For this review, take the finished solid that the model builds, in its own axes (mm). A direction names the side the tool comes from. Give positions to 0.01 mm unless a question says otherwise; leave off trailing zeros. Order: outer loops, then holes, each group sorted by start corner. A loop starts at its lowest first (then second) coordinate and runs counter-clockwise, first axis right, second up. Notation, with made-up numbers: (88, 75.25) -> (122, 75.25) arc R27 cw to (122, 92.25) -> close; hole circle Ø11 at (24.5, 31.25). An arc over 180 degrees is marked (long way). One line per item, written item: value. Start each with the question number.
from build123d import *

# Parameters (mm, degrees)
SKETCH2_R           = 4.2
BOSS_EXTRUDE1_DEPTH = 100
FILLET1_R           = 5


with BuildPart() as part:
    # Sketch2 → Boss-Extrude1 (new body)
    with BuildSketch(Plane.XY):
        with BuildLine():
            Line((15.440624277, -4.881535018), (15.440624277, -0.681535018))
            ThreePointArc((15.440624277, -0.681535018), (3.240624277, 11.518464982), (-8.959375723, -0.681535018))
            Line((-8.959375723, -0.681535018), (-8.959375723, -4.881535018))
            Line((-8.959375723, -4.881535018), (-43.959375723, -4.881535018))
            Line((-43.959375723, -4.881535018), (-43.959375723, -10.881535018))
            Line((-43.959375723, -10.881535018), (50.440624277, -10.881535018))
            Line((50.440624277, -10.881535018), (50.440624277, -4.881535018))
            Line((50.440624277, -4.881535018), (15.440624277, -4.881535018))
        make_face()
        with Locations((3.240624277, -0.681535018)):
            Circle(SKETCH2_R, mode=Mode.SUBTRACT)
    extrude(amount=BOSS_EXTRUDE1_DEPTH)

    # Fillet1
    fillet1_edges = [part.edges().sort_by_distance(p)[0] for p in [
        (-8.959375723, -4.881535018, 50),
        (15.440624277, -4.881535018, 50),
    ]]
    fillet(fillet1_edges, radius=FILLET1_R)


solid = part.part
Q1. Take a section at A-A (x = 0.5). State the section outline as (y, z) points.
Q2. Take a section at B-B (y = 1.75). State the section outline as (x, z) points.
Q3. Mouldability with a two-part tool opening along Y and no side actions: class faces 1 (the cylindrical face through (-0.09, -3.24, 49.3)), 2 (the flat face through (36, -4.882, 49)), 3 (the flat face through (3, -10.882, 49)) as pulls with the +Y half, pulls with the -Y half, needs draft (parallel to the pull), parting line crosses it, or undercut.
Q4. For line 1 along Y through (x, z) = (-36.5, 29.5); line 2 along X through (y, z) = (2, 83); line 3 along X through (y, z) = (1.5, 35.5), list the stretches that pass through material, from the lowest coordinate up.
Q5. For faces 4 (the flat face through (50.441, -8, 49)), 5 (the flat face through (-29, -4.882, 49)), list the 3-axis set-ups (+Z, -Z, +X, -X, +Y, -Y) from which the entire face can be reached by the end or side of a thin tool; tool diameter is ignored.
Q6. Take a section at C-C (x = 35.5). State the section outline as (y, z) points.
Q7. For pin 1 Ø6 at (x, z) = (24, 12) entering from +Y; pin 2 Ø3 at (y, z) = (9, 32) entering from +X; pin 3 Ø12 at (y, z) = (2, 10.5) entering from -X, all flat-tipped, find the tip position at first contact; note any pin that passes through.
Q8. Take a section at D-D (y = 8.5). State the section outline as (x, z) points, and give its area (3 significant figures).
Answers below:
1. outline: (-10.88, 0) -> (-3.86, 0) -> (-3.86, 100) -> (-10.88, 100) -> close; (2.5, 0) -> (11.21, 0) -> (11.21, 100) -> (2.5, 100) -> close
2. outline: (-8.71, 0) -> (-0.18, 0) -> (-0.18, 100) -> (-8.71, 100) -> close; (6.67, 0) -> (15.2, 0) -> (15.2, 100) -> (6.67, 100) -> close
3. face 1: undercut
3. face 2: pulls with the +Y half
3. face 3: pulls with the -Y half
4. line 1: y = -10.88 to -4.88
4. line 2: x = -8.66 to 0.01, 6.47 to 15.14
4. line 3: x = -8.76 to -0.35, 6.83 to 15.24
5. face 4: +Z, -Z, +X, +Y, -Y
5. face 5: +Z, -Z, -X, +Y
6. outline: (-10.88, 0) -> (-4.88, 0) -> (-4.88, 100) -> (-10.88, 100) -> close
7. pin 1: stops at y = -4.88
7. pin 2: stops at x = 12.29
7. pin 3: stops at x = -11.11
8. outline: (-4.79, 0) -> (11.27, 0) -> (11.27, 100) -> (-4.79, 100) -> close
8. area: 1,610 mm²
